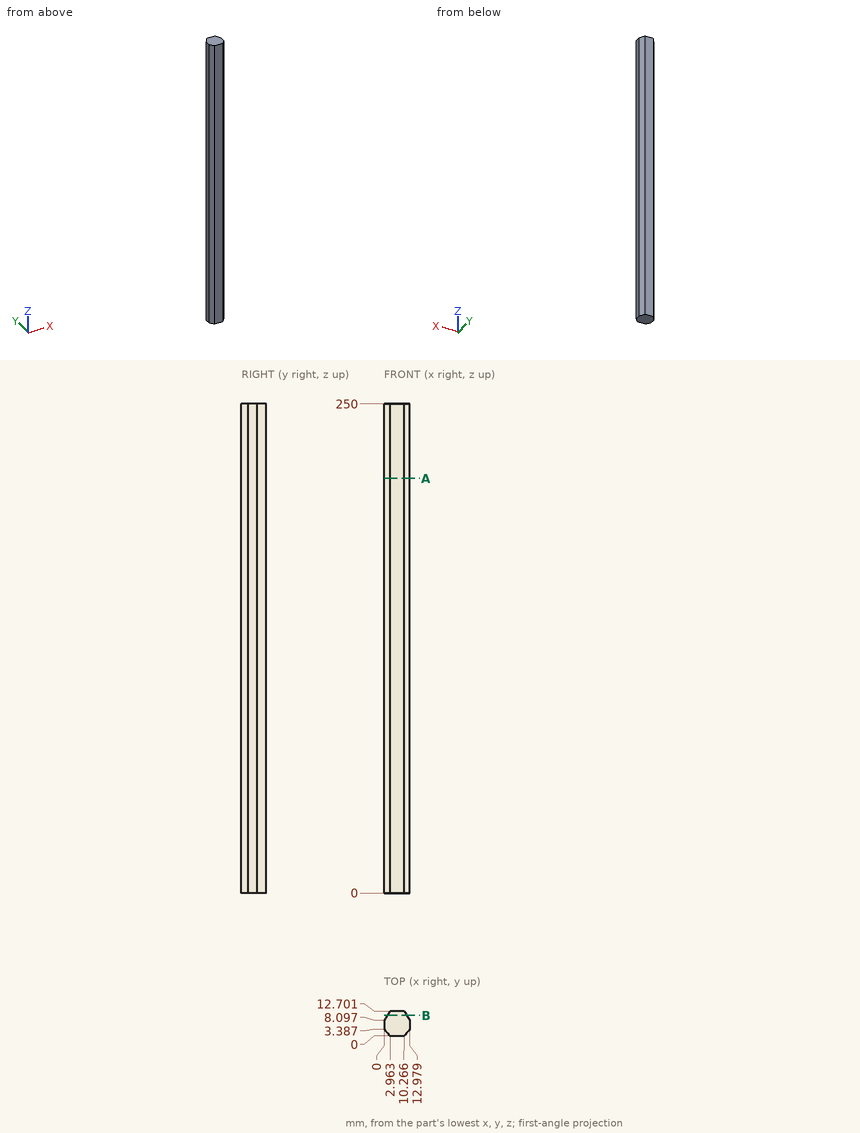
Geometry check sheet. Reference: drawing and pictorial views, mm from the part's lowest x, y, z. Coordinates: 2 decimals unless noted, no trailing zeros. Write each loop counter-clockwise with the first axis right and the second up, starting at its lowest first coordinate (ties: lowest second). Pieces come first, ordered by that corner, then holes.
Item 1: Scan lines: probe 1 along X at (y, z) = (3.25, 146); probe 2 along X at (y, z) = (8.5, 67); probe 3 along Y at (x, z) = (10.5, 99.5) (1 decimal). Record each from-to range of solid material in increasing order.
Numbers:
probe 1: x = 0.12 to 12.87
probe 2: x = 0.26 to 12.74
probe 3: y = 0.3 to 12.3
Item 2: Cross-section at A-A on z = 212. Record the boundary of the cut face in (x, y).
Numbers:
outline: (0, 3.39) - (2.96, 0) - (10.27, 0) - (12.98, 3.39) - (12.98, 8.1) - (10.27, 12.7) - (2.96, 12.7) - (0, 8.1) - close
Item 3: Cross-section at B-B on y = 10.5. Record the boundary of the cut face in (x, z), then the cut area to 3 significant figures.
Numbers:
outline: (1.55, 0) - (11.56, 0) - (11.56, 250) - (1.55, 250) - close
area: 2,500 mm2
